Design review of the part built by this model. Coordinates are the model's own, in mm. Face numbers are marked on the shaded views. Round coordinates to 2 decimals unless told otherwise and drop trailing zeros. Order: outer loops, then holes, each group sorted by start corner. A loop starts at its lowest first (then second) coordinate and runs counter-clockwise, first axis right, second up. Notation, with made-up numbers: (29.5, -12) - (45.5, -12) arc R21 ccw to (45.5, -7) - close; hole circle Ø4 at (12, 48.25). An arc over 180 degrees is marked (long way). Use CSV: the item, a comma, the result in double quotes.
from build123d import *

# Parameters (mm, degrees)
F0_W     = 88.9
F0_H     = 63.5
F1_DEPTH = 25.4


with BuildPart() as f1:
    # F0 (on Front) → F1 (new body)
    with BuildSketch(Plane.XZ):
        Rectangle(F0_W, F0_H)
        with BuildLine():
            ThreePointArc((-25.4, 6.9723), (-29.4500955106, 16.7500955106), (-19.6723, 12.7))
            Line((-19.6723, 12.7), (-5.7277, 12.7))
            ThreePointArc((-5.7277, 12.7), (0, 18.4277), (5.7277, 12.7))
            Line((5.7277, 12.7), (19.6723, 12.7))
            ThreePointArc((19.6723, 12.7), (25.4, 18.4277), (31.1277, 12.7))
            ThreePointArc((31.1277, 12.7), (29.4500955106, 8.6499044894), (25.4, 6.9723))
            Line((25.4, 6.9723), (25.4, -6.9723))
            ThreePointArc((25.4, -6.9723), (29.4500955106, -8.6499044894), (31.1277, -12.7))
            ThreePointArc((31.1277, -12.7), (25.4, -18.4277), (19.6723, -12.7))
            Line((19.6723, -12.7), (5.7277, -12.7))
            ThreePointArc((5.7277, -12.7), (0, -18.4277), (-5.7277, -12.7))
            Line((-5.7277, -12.7), (-19.6723, -12.7))
            ThreePointArc((-19.6723, -12.7), (-29.4500955106, -16.7500955106), (-25.4, -6.9723))
            Line((-25.4, -6.9723), (-25.4, 6.9723))
        make_face(mode=Mode.SUBTRACT)
        with BuildLine():
            Line((-5.7277, 12.7), (-19.6723, 12.7))
            ThreePointArc((-19.6723, 12.7), (-21.3499044894, 8.6499044894), (-25.4, 6.9723))
            Line((-25.4, 6.9723), (-25.4, -6.9723))
            ThreePointArc((-25.4, -6.9723), (-21.3499044894, -8.6499044894), (-19.6723, -12.7))
            Line((-19.6723, -12.7), (-5.7277, -12.7))
            ThreePointArc((-5.7277, -12.7), (0, -6.9723), (5.7277, -12.7))
            Line((5.7277, -12.7), (19.6723, -12.7))
            ThreePointArc((19.6723, -12.7), (21.3499044894, -8.6499044894), (25.4, -6.9723))
            Line((25.4, -6.9723), (25.4, 6.9723))
            ThreePointArc((25.4, 6.9723), (21.3499044894, 8.6499044894), (19.6723, 12.7))
            Line((19.6723, 12.7), (5.7277, 12.7))
            ThreePointArc((5.7277, 12.7), (0, 6.9723), (-5.7277, 12.7))
        make_face()
    extrude(amount=F1_DEPTH)


solid = f1.part
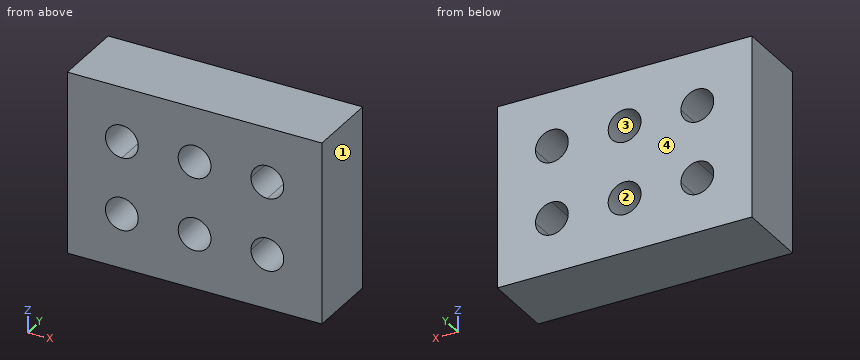
1) We need section C-C (y = -23.25). Give the boundary of the cut face in (x, z), then the cut area to 3 significant figures.
Data:
outline,"(-44.45, -31.75) - (44.45, -31.75) - (44.45, 31.75) - (-44.45, 31.75) - close; hole circle Ø11.46 at (-25.4, -12.7); hole circle Ø11.46 at (-25.4, 12.7); hole circle Ø11.46 at (0, -12.7); hole circle Ø11.46 at (0, 12.7); hole circle Ø11.46 at (25.4, -12.7); hole circle Ø11.46 at (25.4, 12.7)"
area,"5,030 mm2"
2) The part is to be moulded in two halves that separate along X. For the marked faces 1, 2, 3 and 4, say which applies: +X half, -X half, draft (parallel to the pull), parting line (faces both ways), or undercut.
Data:
face 1,"+X half"
face 2,"undercut"
face 3,"undercut"
face 4,"draft"
3) To check wall thickness, follow L1, parallel to Z at x = 0, y = -6.5; L2, parallel to X at y = -5.75, z = 12.7; L3, parallel to X at y = -9, z = -15. State the ranges of each line that lie inside material, in increasing order. Write a range as from..to.
Data:
L1,"z = -31.75..-18.43, -6.97..6.97, 18.43..31.75"
L2,"x = -44.45..-31.13, -19.67..-5.73, 5.73..19.67, 31.13..44.45"
L3,"x = -44.45..-30.65, -20.15..-5.25, 5.25..20.15, 30.65..44.45"
4) We need section D-D (z = 11). Give the boundary of the cut face in (x, y).
Data:
outline,"(-44.45, -25.4) - (-30.87, -25.4) - (-30.87, 0) - (-44.45, 0) - close; (-19.93, -25.4) - (-5.47, -25.4) - (-5.47, 0) - (-19.93, 0) - close; (5.47, -25.4) - (19.93, -25.4) - (19.93, 0) - (5.47, 0) - close; (30.87, -25.4) - (44.45, -25.4) - (44.45, 0) - (30.87, 0) - close"
5) We need section A-A (x = 0). Give the boundary of the cut face in (y, z), then the cut area to 3 significant figures.
Data:
outline,"(-25.4, -31.75) - (0, -31.75) - (0, -18.43) - (-25.4, -18.43) - close; (-25.4, -6.97) - (0, -6.97) - (0, 6.97) - (-25.4, 6.97) - close; (-25.4, 18.43) - (0, 18.43) - (0, 31.75) - (-25.4, 31.75) - close"
area,"1,030 mm2"
6) We need section B-B (z = -16). Give the boundary of the cut face in (x, y), then the cut area to 3 significant figures.
Data:
outline,"(-44.45, -25.4) - (-30.08, -25.4) - (-30.08, 0) - (-44.45, 0) - close; (-20.72, -25.4) - (-4.68, -25.4) - (-4.68, 0) - (-20.72, 0) - close; (4.68, -25.4) - (20.72, -25.4) - (20.72, 0) - (4.68, 0) - close; (30.08, -25.4) - (44.45, -25.4) - (44.45, 0) - (30.08, 0) - close"
area,"1,540 mm2"
